Verification items for the finished model (mm, model axes). Face numbers are marked on the shaded views. A direction names the side the tool comes from. Round coordinates to 2 decimals unless told otherwise and drop trailing zeros. Loops run counter-clockwise (first coordinate to the right, second up) from the corner with the lowest first, then second, coordinate; pieces in that order, holes last. Notation, with made-up numbers: M 7,51 L 28,51 A22 cw 28,82 Z; hole C -8.75,71.5 d7. An arc over 180 degrees is marked long. Answer as CSV lines item,"result".
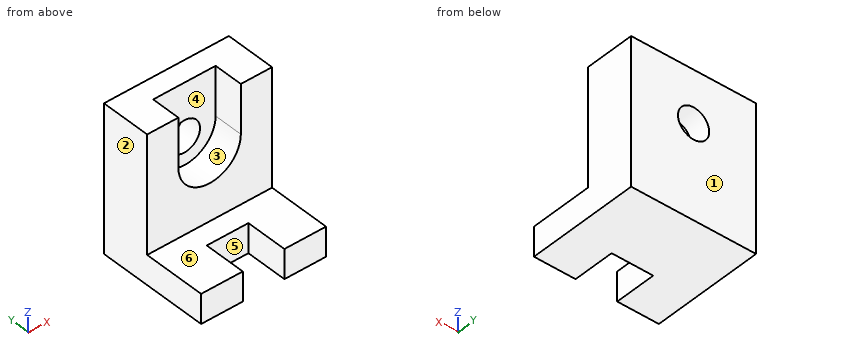
```python
from build123d import *

# Parameters (mm, degrees)
F0_W      = 60
F0_H      = 70
F1_DEPTH  = 24
F3_DEPTH  = 14
F4_R      = 7.5
F5_DEPTH  = 24.001
F6_W      = 60
F6_H      = 14
F7_DEPTH  = 30
F10_DEPTH = 20
F11_DEPTH = 0.1359600746


with BuildPart() as f1:
    # F0 (on Front) → F1 (new body)
    with BuildSketch(Plane.XZ):
        Rectangle(F0_W, F0_H)
    extrude(amount=F1_DEPTH)

    # F2 (on face) → F3 (cut)
    with BuildSketch(Plane.XZ.offset(24)):
        with BuildLine():
            Line((15, 35), (-15, 35))
            Line((-15, 35), (-15, 11.6464606471))
            ThreePointArc((-15, 11.6464606471), (0, -3.3535393529), (15, 11.6464606471))
            Line((15, 11.6464606471), (15, 35))
        make_face()
    extrude(amount=-F3_DEPTH, mode=Mode.SUBTRACT)

    # F4 (on face) → F5 (cut, through all)
    with BuildSketch(Plane(origin=(0, 0, 0), x_dir=(-1, 0, 0), z_dir=(0, 1, 0))):
        with Locations((0, 10)):
            Circle(F4_R)
    extrude(amount=-F5_DEPTH, mode=Mode.SUBTRACT)

    # F6 (on face) → F7 (join)
    with BuildSketch(Plane.XZ.offset(24)):
        with Locations((0, -28)):
            Rectangle(F6_W, F6_H)
    extrude(amount=F7_DEPTH)

    # F9 (on face) → F10 (cut)
    with BuildSketch(Plane.XZ.offset(54)):
        Polygon((10, -21), (-9.999969219, -21), (-9.999969219, -34.9001288414), (10, -34.9352178571), align=None)
    extrude(amount=-F10_DEPTH, mode=Mode.SUBTRACT)

    # F11 (cut, through all): a face of the model
    f11_faces = [f1.faces().sort_by_distance(p)[0] for p in [
        (1.53905e-05, -44, -34.9176733492),
    ]]
    extrude(f11_faces, amount=-F11_DEPTH, mode=Mode.SUBTRACT)


solid = f1.part
```
1) Section check D-D (y = -13). Record the cut outline in (x, z), plus the area to 3 significant figures.
Here are the results:
outline,"M -30,-35 L 30,-35 L 30,35 L 15,35 L 15,11.65 A15 cw -15,11.65 L -15,35 L -30,35 Z"
area,"3,150 mm^2"
2) Section check C-C (z = 10). Record the cut outline in (x, y), plus the area to 3 significant figures.
Here are the results:
outline,"M -30,-24 L -14.91,-24 L -14.91,-10 L -7.5,-10 L -7.5,0 L -30,0 Z; M 7.5,-10 L 14.91,-10 L 14.91,-24 L 30,-24 L 30,0 L 7.5,0 Z"
area,"873 mm^2"
3) Material ranges on probe 1 along Z at (x, y) = (0, -4.25); probe 2 along X at (y, z) = (-42, -24.5); probe 3 along Y at (x, z) = (23.5, 29), recorded low to high.
Here are the results:
probe 1,"z = -35 to 2.5, 17.5 to 35"
probe 2,"x = -30 to -10, 10 to 30"
probe 3,"y = -24 to 0"
4) Section check B-B (x = 0). Record the cut outline in (y, z), plus the area to 3 significant figures.
Here are the results:
outline,"M -34,-35 L 0,-35 L 0,2.5 L -10,2.5 L -10,-3.35 L -24,-3.35 L -24,-21 L -34,-21 Z; M -10,17.5 L 0,17.5 L 0,35 L -10,35 Z"
area,"1,130 mm^2"
5) Section check A-A (y = -47.5). Record the cut outline in (x, z).
Here are the results:
outline,"M -30,-35 L -10,-35 L -10,-34.9 L -10,-21 L -30,-21 Z; M 10,-35 L 30,-35 L 30,-21 L 10,-21 L 10,-34.94 Z"
6) Draft check along X on the marked faces 1, 2 and 3. Enter one of: +X half, -X half, draft (parallel to the pull), parting line (faces both ways), or undercut.
Here are the results:
face 1,"draft"
face 2,"-X half"
face 3,"undercut"
7) Go/stop test with flat-tipped pins: pin 1 (13.5 mm diameter, centred on x = 0, z = 10, fed in from -Y); pin 2 (9 mm diameter, centred on x = 2.5, z = 19.5, fed in from -Y); pin 3 (10 mm diameter, centred on x = 15, z = -2, fed in from -Y); pin 4 (2 mm diameter, centred on x = -9.5, y = -41.5, fed in from +Z). Record where each tip stops, or that it passes through.
Here are the results:
pin 1,"passes through"
pin 2,"stops at y = -10"
pin 3,"stops at y = -24"
pin 4,"stops at z = -21"
8) Set-up check for the marked faces 4, 5 and 6: record each of +Z, -Z, +X, -X, +Y, -Y from which the full face is reachable in a straight line by a thin tool's end or side.
Here are the results:
face 4,"+Z, -Y"
face 5,"+Z, -Z, -Y"
face 6,"+Z, +X, -X, -Y"
